Design review of the part built by this model. Coordinates are the model's own, in mm. Coordinates: 2 decimals unless noted, no trailing zeros. Write each loop counter-clockwise with the first axis right and the second up, starting at its lowest first coordinate (ties: lowest second). Pieces come first, ordered by that corner, then holes. Notation, with made-up numbers: (-13.5, 39.5) -> (17.5, 39.5) arc R15 cw to (17.5, 51.5) -> close; hole circle Ø8 at (60, -28). An arc over 180 degrees is marked (long way). Answer in a Markdown table with one row per item. Add a question column.
Item 1: Take a section at B-B, the plane x = 7.15. Write out the cut boundary in (y, z).
Item 2: Take a section at A-A, the plane z = -3.6. Write out the cut boundary in (x, y), and give its area (3 significant figures).
Item 3: To check wall thickness, follow line 1 (X direction, y = -2, z = -18); line 2 (Z direction, x = 7.15, y = -1.35); line 3 (Z direction, x = -7.15, y = -2.2). State the ranges of each line that lie inside material, in increasing order.
Item 4: Take a section at C-C, the plane y = -2.1. Write out the cut boundary in (x, z).
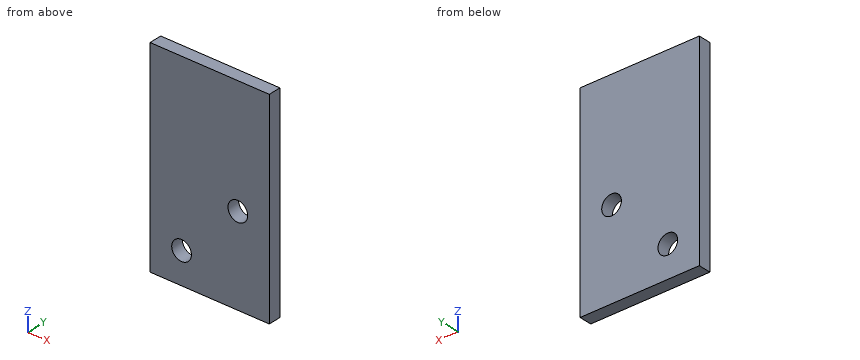
from build123d import *

# Parameters (mm, degrees)
SKETCH1_W           = 30.3
SKETCH1_H           = 52
BOSS_EXTRUDE1_DEPTH = 3.2
M6_TAPPED_HOLE1_D   = 5


with BuildPart() as part:
    # Sketch1 → Boss-Extrude1 (new body)
    with BuildSketch(Plane(origin=(0, 0, 0), x_dir=(1, 0, 0), z_dir=(0, 1, 0))):
        Rectangle(SKETCH1_W, SKETCH1_H)
    extrude(amount=-BOSS_EXTRUDE1_DEPTH)

    # M6 Tapped Hole1 (through all)
    with Locations(Plane(origin=(0, 0, 0), x_dir=(1, 0, 0), z_dir=(0, 1, 0))):
        with Locations((-7.15, 18), (7.15, 3.6)):
            Hole(M6_TAPPED_HOLE1_D / 2)


solid = part.part
Answers:
| question | item | result |
|---|---|---|
| 1 | outline | (-3.2, -26) -> (0, -26) -> (0, -6.1) -> (-3.2, -6.1) -> close; (-3.2, -1.1) -> (0, -1.1) -> (0, 26) -> (-3.2, 26) -> close |
| 2 | outline | (-15.15, -3.2) -> (4.65, -3.2) -> (4.65, 0) -> (-15.15, 0) -> close; (9.65, -3.2) -> (15.15, -3.2) -> (15.15, 0) -> (9.65, 0) -> close |
| 2 | area | 81.0 mm^2 |
| 3 | line 1 | x = -15.15 to -9.65, -4.65 to 15.15 |
| 3 | line 2 | z = -26 to -6.1, -1.1 to 26 |
| 3 | line 3 | z = -26 to -20.5, -15.5 to 26 |
| 4 | outline | (-15.15, -26) -> (15.15, -26) -> (15.15, 26) -> (-15.15, 26) -> close; hole circle Ø5 at (-7.15, -18); hole circle Ø5 at (7.15, -3.6) |
